Part print with two shaded views. Sizes in mm from the minimum x, y, z corner. Give positions to 0.01 mm unless a question says otherwise; leave off trailing zeros. Write each loop counter-clockwise with the first axis right and the second up, starting at its lowest first coordinate (ties: lowest second). Pieces come first, ordered by that corner, then holes. Notation, with made-up numbers: M -4.5,-35.5 L 6.5,-35.5 A9 cw 6.5,-22.5 Z; hole C 52.25,-26 d6. An arc over 180 degrees is marked long. One line per item, written item: value. Start each with the question number.
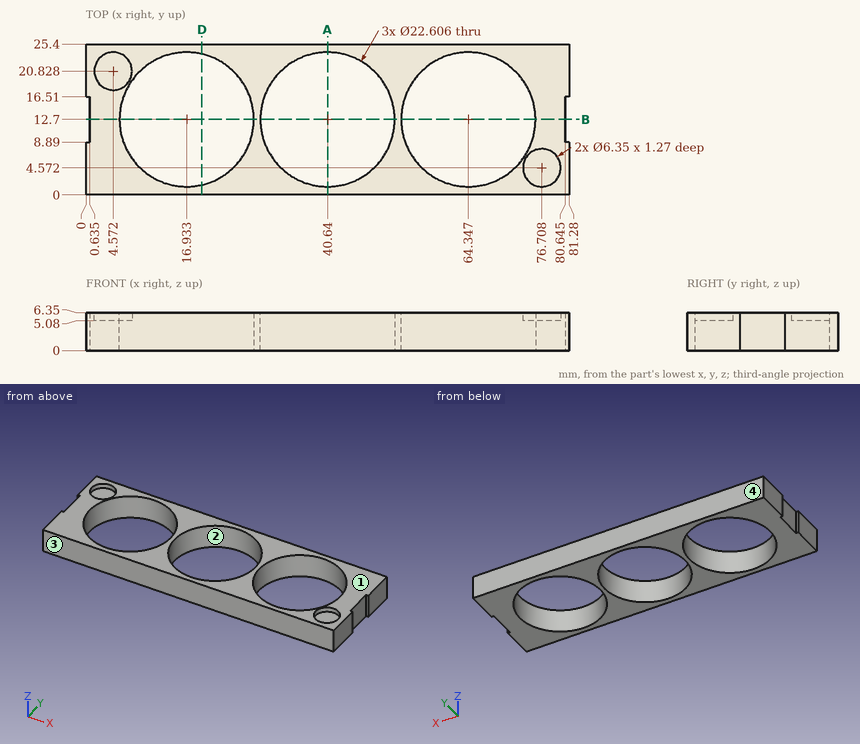
1) Band-saw the part on D-D (x = 19.5). List the corners of the cut face in (y, z), then the cut area to 3 significant figures.
2) Mould opens along Y. For the marked faces 1, 2, 3 and 4 say: released by +Y, released by -Y, zero draft, split by the parting line, or undercut.
3) Drop flat-ended pins along their axis: P1, Ø5.5, axis at x = 76.708, y = 4.572, coming from the +Z side; P2, Ø12, axis at x = 49, y = 8.5, coming from the +Z side; P3, Ø1.9, axis at y = 12.5, z = 3, coming from the +X side (3 decimals). Give the stop position or say it passes through.
4) Band-saw the part on A-A (x = 40.64). List the corners of the cut face in (y, z).
5) Probe line 1 along X through (y, z) = (13, 6) (1 decimal); line 2 along Y through (x, z) = (17, 0.75); line 3 along X through (y, z) = (5, 2.25) (1 decimal). List the from-to ranges inside material, lowest first. Write a range as from..to.
6) Band-saw the part on B-B (y = 12.7). Count the separate pieces of the cut face and the enclosed holes in it.
Model answer:
1. outline: M 0,0 L 1.69,0 L 1.69,6.35 L 0,6.35 Z; M 23.71,0 L 25.4,0 L 25.4,6.35 L 23.71,6.35 Z
1. area: 21.5 mm²
2. face 1: zero draft
2. face 2: undercut
2. face 3: released by -Y
2. face 4: released by +Y
3. P1: stops at z = 5.08
3. P2: stops at z = 6.35
3. P3: stops at x = 80.645
4. outline: M 0,0 L 1.4,0 L 1.4,6.35 L 0,6.35 Z; M 24,0 L 25.4,0 L 25.4,6.35 L 24,6.35 Z
5. line 1: x = 0.6..5.6, 28.2..29.3, 51.9..53, 75.6..80.6
5. line 2: y = 0..1.4, 24..25.4
5. line 3: x = 0..8.7, 25.2..32.4, 48.9..56.1, 72.6..81.3
6. separate pieces: 4
6. enclosed holes: 0
